Autodesk Inventor part; units mm, degrees
ref_plane "YZ Plane" through (0, 0, 0) normal (1, 0, 0) x (0, 1, 0)
ref_plane "XZ Plane" through (0, 0, 0) normal (0, 1, 0) x (-1, 0, 0)
ref_plane "XY Plane" through (0, 0, 0) normal (0, 0, 1) x (1, 0, 0)
sketch "Sketch1" plane through (0, 0, 0) normal (0, 0, 1) x (1, 0, 0)
  line L0 (-17.2121, 7.0196) -> (12.7879, 7.0196)
  line L1 (12.7879, 7.0196) -> (12.7879, -22.9804)
  line L2 (12.7879, -22.9804) -> (-17.2121, -22.9804)
  line L3 (-17.2121, -22.9804) -> (-17.2121, 7.0196)
  line L4 (11.0879, -22.9804) -> (11.0879, 7.0196)
  line L5 (-17.2121, 5.3196) -> (12.7879, 5.3196)
  line L6 (-15.5121, 7.0196) -> (-15.5121, -22.9804)
  line L7 (-17.2121, -21.2804) -> (12.7879, -21.2804)
  point P0 (-15.5121, -21.2804)
  point P1 (11.0879, -21.2804)
  point P2 (11.0879, 5.3196)
  point P3 (-15.5121, 5.3196)
  dimension "d1" = 30
  dimension "d2" = 30
  dimension "d3" = 1.7
  dimension "d4" = 1.7
  dimension "d5" = 1.7
  dimension "d6" = 1.7
extrude "Extrusion1" add sketch "Sketch1" against normal blind 255
extrude "Extrusion2" cut sketch "Sketch1" against normal blind 430 contours L5 L4 L7 L6
properties part number "Cablecanal Ranurado 30x30 L=255 mm" material "PPS Plastic"
Build history of the part. All positions in model axes, mm. A direction names the side the tool comes from. Round coordinates to 2 decimals unless told otherwise and drop trailing zeros. Loops run counter-clockwise (first coordinate to the right, second up) from the corner with the lowest first, then second, coordinate; pieces in that order, holes last. Notation, with made-up numbers: (84, 81) -> (115, 81) arc R20 ccw to (115, 107) -> close; hole circle Ø7 at (63, 66.5). An arc over 180 degrees is marked (long way). Use CSV: the item, a comma, the result in double quotes. Start each with the question number.
Q1. Which spindle directions (+Z, -Z, +X, -X, +Y, -Y) get a long thin tool onto all of the face, cutting with end or side? Do faces 1 (the face through (-17.212, -8, -126)), 2 (the face through (11.088, -8, -126)). Say none if no direction does.
Q2. Saw through at C-C on z = -71. Give the cut face in (x, y), and give its area (3 significant figures).
Q3. Saw through at A-A on x = -9. Give the cut face in (y, z).
Q4. Drill centre lines: L1, parallel to Y at x = -8.75, z = -38.5; L2, parallel to X at y = 3.75, z = -241.5. Where is each one in solid material? Low to high.
Q5. Mould opens along Y. For faces 3 (the face through (-16, -6, -255)), 4 (the face through (-2, -22.98, -126)), 5 (the face through (-2, -21.28, -126)) say: +Y half, -Y half, draft (parallel to the pull), parting line (faces both ways), or undercut.
Q6. Saw through at B-B on y = -13. Give the cut face in (x, z), and give its area (3 significant figures).
Solutions:
1,face 1,"+Z, -Z, -X, +Y, -Y"
1,face 2,"+Z, -Z"
2,outline,"(-17.21, -22.98) -> (12.79, -22.98) -> (12.79, 7.02) -> (-17.21, 7.02) -> close; hole (-15.51, -21.28) -> (11.09, -21.28) -> (11.09, 5.32) -> (-15.51, 5.32) -> close"
2,area,"192 mm^2"
3,outline,"(-22.98, -255) -> (-21.28, -255) -> (-21.28, 0) -> (-22.98, 0) -> close; (5.32, -255) -> (7.02, -255) -> (7.02, 0) -> (5.32, 0) -> close"
4,L1,"y = -22.98 to -21.28, 5.32 to 7.02"
4,L2,"x = -17.21 to -15.51, 11.09 to 12.79"
5,face 3,"draft"
5,face 4,"-Y half"
5,face 5,"undercut"
6,outline,"(-17.21, -255) -> (-15.51, -255) -> (-15.51, 0) -> (-17.21, 0) -> close; (11.09, -255) -> (12.79, -255) -> (12.79, 0) -> (11.09, 0) -> close"
6,area,"867 mm^2"
